Check sheet for the drawn part. Datum: minimum x, y, z corner. Units: mm. A direction names the side the tool comes from. Round coordinates to 2 decimals unless told otherwise and drop trailing zeros. Write each loop counter-clockwise with the first axis right and the second up, starting at its lowest first coordinate (ties: lowest second). Pieces come first, ordered by that corner, then holes. Notation, with made-up numbers: M 83,88.25 L 100,88.25 A17 cw 100,94.25 Z; hole C -20,67 d2. An arc over 180 degrees is marked long. Answer in a Markdown table with one row per item. Add a question column.
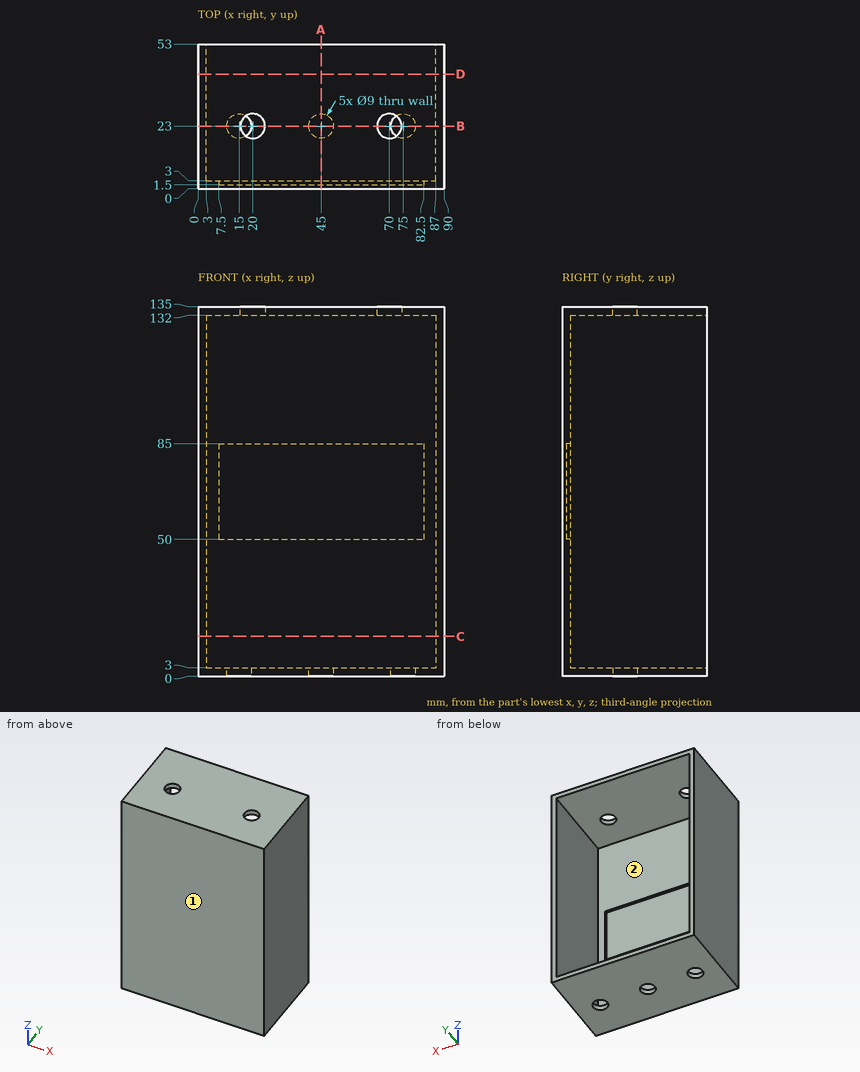
Item 1: Section check B-B, the plane y = 23. Record the boundary of the cut face in (x, z).
Item 2: Gauge pin test, flat ends, axial feed: pin 1 Ø25 at (x, z) = (35.5, 85.5) entering from +Y; pin 2 Ø1 at (x, z) = (19, 55) entering from -Y; pin 3 Ø17.5 at (x, z) = (53, 59.5) entering from +Y. Record the tip position at first contact, or that the pin passes through.
Item 3: Access from +Z, -Z, +X, -X, +Y, -Y to the whole of each face (thin tool, end or side, straight path). Record for the marked faces 1 and 2.
Item 4: Scan lines: probe 1 along Z at (x, y) = (6.5, 12); probe 2 along Y at (x, z) = (45, 1.5); probe 3 along X at (y, z) = (18.5, 85.5). Record each from-to range of solid material in increasing order. Write a range as from..to.
Item 5: Section check A-A, the plane x = 45. Record the boundary of the cut face in (y, z).
Item 6: Section check D-D, the plane y = 42. Record the boundary of the cut face in (x, z).
Item 7: Section check C-C, the plane z = 14.5. Record the boundary of the cut face in (x, y).
Result sheet:
| question | item | result |
|---|---|---|
| 1 | outline | M 0,0 L 10.5,0 L 10.5,3 L 3,3 L 3,132 L 15.5,132 L 15.5,135 L 0,135 Z; M 19.5,0 L 40.5,0 L 40.5,3 L 19.5,3 Z; M 24.5,132 L 65.5,132 L 65.5,135 L 24.5,135 Z; M 49.5,0 L 70.5,0 L 70.5,3 L 49.5,3 Z; M 74.5,132 L 87,132 L 87,3 L 79.5,3 L 79.5,0 L 90,0 L 90,135 L 74.5,135 Z |
| 2 | pin 1 | stops at y = 3 |
| 2 | pin 2 | stops at y = 0 |
| 2 | pin 3 | stops at y = 1.5 |
| 3 | face 1 | +Z, -Z, +X, -X, -Y |
| 3 | face 2 | +Y |
| 4 | probe 1 | z = 0..3, 132..135 |
| 4 | probe 2 | y = 0..18.5, 27.5..53 |
| 4 | probe 3 | x = 0..3, 87..90 |
| 5 | outline | M 0,0 L 18.5,0 L 18.5,3 L 3,3 L 3,50 L 1.5,50 L 1.5,85 L 3,85 L 3,132 L 53,132 L 53,135 L 0,135 Z; M 27.5,0 L 53,0 L 53,3 L 27.5,3 Z |
| 6 | outline | M 0,0 L 90,0 L 90,135 L 0,135 Z; hole M 3,3 L 87,3 L 87,132 L 3,132 Z |
| 7 | outline | M 0,0 L 90,0 L 90,53 L 87,53 L 87,3 L 3,3 L 3,53 L 0,53 Z |
